The listing builds one solid part. Answer for the finished solid, in the listing's coordinates (mm). Face numbers are marked on the shaded views. A direction names the side the tool comes from. Coordinates: 2 decimals unless noted, no trailing zeros. Order: outer loops, then holes, each group sorted by start corner. A loop starts at its lowest first (then second) coordinate and runs counter-clockwise, first axis right, second up. Notation, with made-up numbers: (44.5, -28.75) -> (69.5, -28.75) arc R27 cw to (69.5, -4.75) -> close; hole circle Ø2 at (0.25, 86.5). An arc over 180 degrees is marked (long way). Write item = value, one per line.
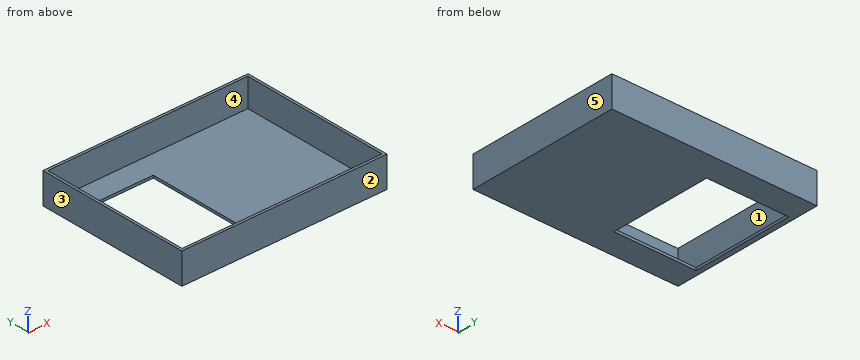
from build123d import *

# Parameters (mm, degrees)
F0_W     = 508
F0_H     = 381
F1_DEPTH = 76.2
F2_W     = 203.2
F2_H     = 254
F3_DEPTH = 76.2
F4_T     = -6.35
F5_W     = 215.9
F5_H     = 266.7
F5_W_2   = 203.2
F5_H_2   = 254
F6_DEPTH = 69.85


# Not quite as in the source:
# - a shell that OpenCascade refuses in one call is made with other operations: the cavity is built on its own and cut out


with BuildPart() as f1:
    # F0 (on Top) → F1 (new body)
    with BuildSketch(Plane.XY):
        Rectangle(F0_W, F0_H)
    extrude(amount=F1_DEPTH)

    # F2 (on face) → F3 (cut, through all)
    with BuildSketch(Plane.XY.offset(76.2)):
        with Locations((-139.7, 0)):
            Rectangle(F2_W, F2_H)
    extrude(amount=-F3_DEPTH, mode=Mode.SUBTRACT)

    # F4: a shell. OpenCascade refuses it in one call, so the cavity is built on its own and cut out:
    # the body offset inwards by the wall thickness, plus a prism from it out through each open face.
    f4_core = offset(f1.part, amount=F4_T, kind=Kind.INTERSECTION, mode=Mode.PRIVATE)
    f4_exits = [f4_core.faces().sort_by_distance(p)[0] for p in [
        (64.435271, 0, 69.85),
    ]]
    add(f4_core, mode=Mode.SUBTRACT)
    extrude(f4_exits, amount=-F4_T, mode=Mode.SUBTRACT)

    # F5 (on face) → F6 (cut)
    with BuildSketch(Plane.XY.offset(76.2)):
        with Locations((-139.7, 0)):
            Rectangle(F5_W, F5_H)
        with Locations((-139.7, 0)):
            Rectangle(F5_W_2, F5_H_2, mode=Mode.SUBTRACT)
    extrude(amount=-F6_DEPTH, mode=Mode.SUBTRACT)


solid = f1.part
Q1. Section C-C, the plane z = 48.5 is taken. Give the vertices of the cut face in (x, y).
The answers:
outline = (-254, -190.5) -> (254, -190.5) -> (254, 190.5) -> (-254, 190.5) -> close; hole (-247.65, -184.15) -> (247.65, -184.15) -> (247.65, 184.15) -> (-247.65, 184.15) -> close
Q2. The mould has two halves that part along X. Classify the marked faces 3, 4 and 5: released by +X, released by -X, zero draft, split by the parting line, or undercut.
The answers:
face_3 = released by -X
face_4 = undercut
face_5 = released by +X
Q3. Section A-A, the plane x = -77 is taken. Give the vertices of the cut face in (y, z).
The answers:
outline = (-190.5, 0) -> (-127, 0) -> (-127, 6.35) -> (-184.15, 6.35) -> (-184.15, 76.2) -> (-190.5, 76.2) -> close; (127, 0) -> (190.5, 0) -> (190.5, 76.2) -> (184.15, 76.2) -> (184.15, 6.35) -> (127, 6.35) -> close
Q4. Section D-D, the plane y = -161 is taken. Give the vertices of the cut face in (x, z), plus the area to 3 significant figures.
The answers:
outline = (-254, 0) -> (254, 0) -> (254, 76.2) -> (247.65, 76.2) -> (247.65, 6.35) -> (-247.65, 6.35) -> (-247.65, 76.2) -> (-254, 76.2) -> close
area = 4,110 mm2
Q5. A tool of negligible diameter and unlimited length cuts with its end or side. For the marked faces 1 and 2, from which of +Z, -Z, +X, -X, +Y, -Y can it reach the whole face along a straight path? Write none if from no direction.
The answers:
face_1 = +Z
face_2 = +Z, -Z, +X, -X, -Y
Q6. This flat-tipped pin is pushed along its axis until it touches: pin 1 Ø12 at (x, y) = (-112.5, -124.5) entering from -Z. Where does it stop, or does it pass through?
The answers:
pin_1 = 0
Q7. Section B-B, the plane y = 86.5 is taken. Give the vertices of the cut face in (x, z), plus the area to 3 significant figures.
The answers:
outline = (-254, 0) -> (-241.3, 0) -> (-241.3, 6.35) -> (-247.65, 6.35) -> (-247.65, 76.2) -> (-254, 76.2) -> close; (-38.1, 0) -> (254, 0) -> (254, 76.2) -> (247.65, 76.2) -> (247.65, 6.35) -> (-38.1, 6.35) -> close
area = 2,820 mm2
Q8. Find the intervals of material crossed by line 1 along X through (y, z) = (169.5, 38.5); line 2 along Y through (x, z) = (-147, 47), in increasing order.
The answers:
line_1 = -254 to -247.65, 247.65 to 254
line_2 = -190.5 to -184.15, 184.15 to 190.5
